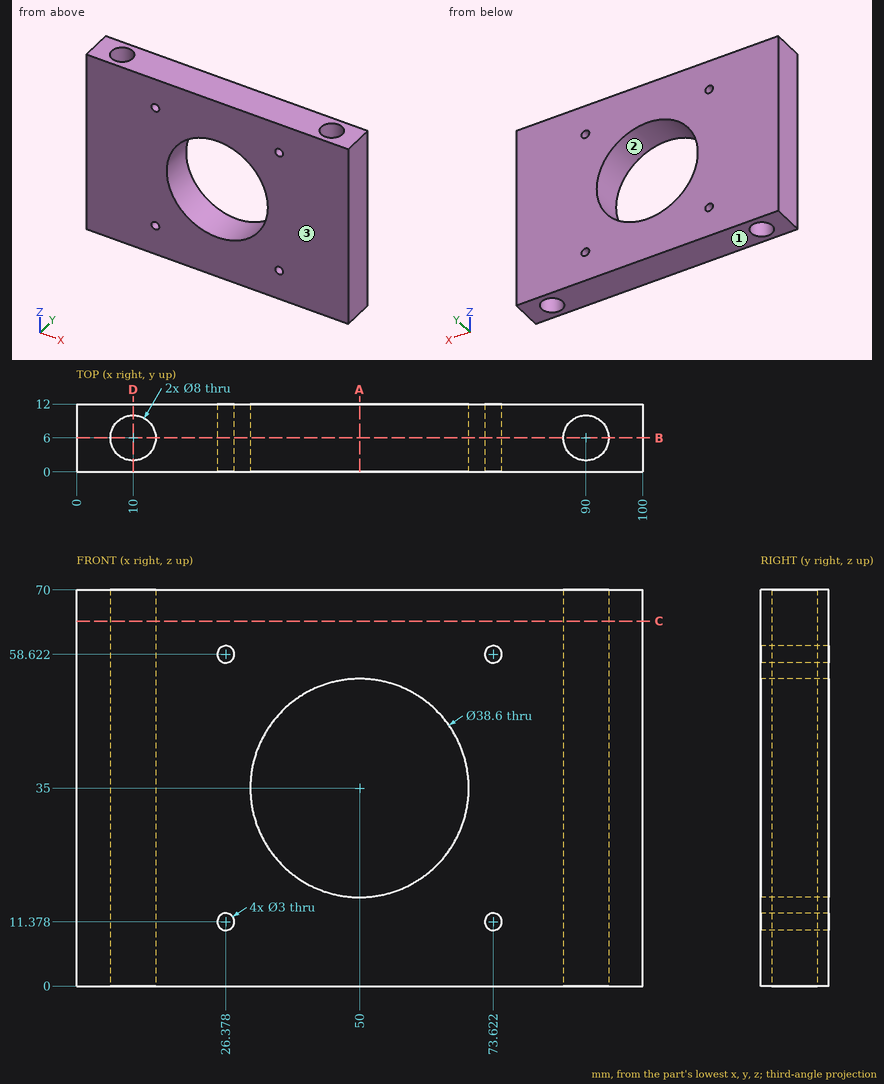
Part print with two shaded views. Sizes in mm from the minimum x, y, z corner. Coordinates: 2 decimals unless noted, no trailing zeros. Order: outer loops, then holes, each group sorted by start corner. A loop starts at its lowest first (then second) coordinate and runs counter-clockwise, first axis right, second up. Notation, with made-up numbers: M 23,49.25 L 78,49.25 A18 ccw 78,76.25 Z; hole C -8,78.25 d2. An arc over 180 degrees is marked long. Use a Markdown table: item, result.
(1) Cut at D-D on x = 10. Write the cut outline in (y, z).
A:
| item | result |
|---|---|
| outline | M 0,0 L 2,0 L 2,70 L 0,70 Z; M 10,0 L 12,0 L 12,70 L 10,70 Z |
(2) Cut at A-A on x = 50. Write the cut outline in (y, z).
A:
| item | result |
|---|---|
| outline | M 0,0 L 12,0 L 12,15.7 L 0,15.7 Z; M 0,54.3 L 12,54.3 L 12,70 L 0,70 Z |
(3) Cut at C-C on z = 64.5. Write the cut outline in (x, y).
A:
| item | result |
|---|---|
| outline | M 0,0 L 100,0 L 100,12 L 0,12 Z; hole C 10,6 d8; hole C 90,6 d8 |
(4) Probe L1, parallel to X at y = 6.25, z = 18.5; L2, parallel to X at y = 7.75, z = 10.5; L3, parallel to X at y = 8, z = 65. List the from-to ranges inside material, lowest first.
A:
| item | result |
|---|---|
| L1 | x = 0 to 6.01, 13.99 to 39.99, 60.01 to 86.01, 93.99 to 100 |
| L2 | x = 0 to 6.4, 13.6 to 25.16, 27.59 to 72.41, 74.84 to 86.4, 93.6 to 100 |
| L3 | x = 0 to 6.54, 13.46 to 86.54, 93.46 to 100 |
(5) Cut at B-B on y = 6. Write the cut outline in (x, z), then the cut area to 3 significant figures.
A:
| item | result |
|---|---|
| outline | M 0,0 L 6,0 L 6,70 L 0,70 Z; M 14,0 L 86,0 L 86,70 L 14,70 Z; M 94,0 L 100,0 L 100,70 L 94,70 Z; hole C 26.38,11.38 d3; hole C 26.38,58.62 d3; hole C 50,35 d38.6; hole C 73.62,11.38 d3; hole C 73.62,58.62 d3 |
| area | 4,680 mm^2 |
(6) Pull direction Z, two halves, no side cores. Call the marked faces 1, 2 and 3: released by +Z, released by -Z, zero draft, split by the parting line, or undercut.
A:
| item | result |
|---|---|
| face 1 | released by -Z |
| face 2 | undercut |
| face 3 | zero draft |
(7) Flat gauge pins, fed straight in: pin 1 (6.5 mm diameter, centred on x = 10, y = 6, fed in from +Z); pin 2 (3.5 mm diameter, centred on x = 73.622, z = 58.622, fed in from -Y). Where does each tip first touch, or does it go through?
A:
| item | result |
|---|---|
| pin 1 | passes through |
| pin 2 | stops at y = 0 |
